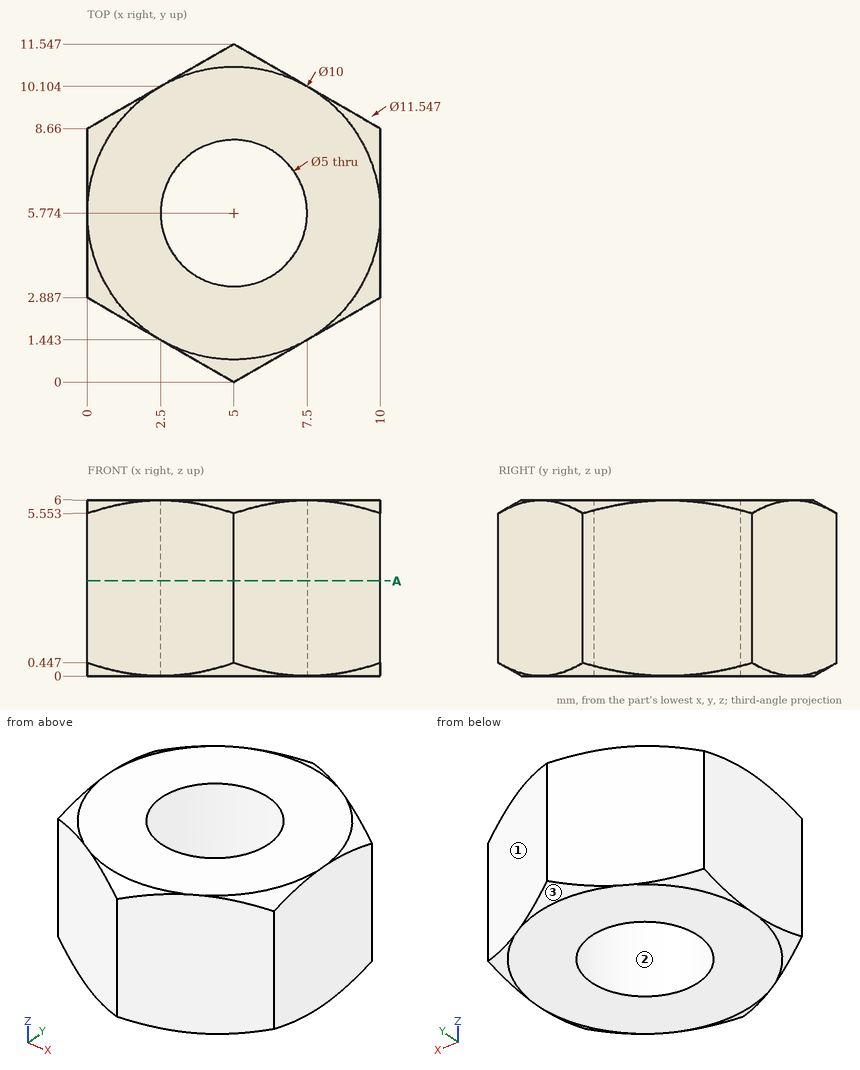
Drawing for the job (mm, zero at the part's lowest x, y, z). Give positions to 0.01 mm unless a question says otherwise; leave off trailing zeros. Write each loop counter-clockwise with the first axis right and the second up, starting at its lowest first coordinate (ties: lowest second). Pieces come first, ordered by that corner, then holes. Notation, with made-up numbers: (-23.5, 6.5) -> (31.5, 6.5) arc R20 cw to (31.5, 16.5) -> close; hole circle Ø11 at (-8.5, 11). An arc over 180 degrees is marked (long way). Put each result on its own line as item: value. Start each with the question number.
Item 1: Wall check: L1, parallel to X at y = 5.75, z = 2.2; L2, parallel to Y at x = 4.25, z = 2.25 (1 decimal); L3, parallel to Y at x = 3.75, z = 1.2 (1 decimal). Give the ranges that are in metal, low to high. Write a range as [from, to].
Item 2: Pull direction X, two halves, no side cores. Call the marked faces 1, 2 and 3: pulls with the +X half, pulls with the -X half, needs draft (parallel to the pull), parting line crosses it, or undercut.
Item 3: Cut at A-A (z = 3.25). List the corners of the cut face in (x, y).
Item 4: Pin check, flat tips, straight feed: pin 1 Ø1 at (x, z) = (8, 3) entering from +Y (1 decimal); pin 2 Ø3 at (x, z) = (8.5, 4.5) entering from -Y (1 decimal). Stop position of each tip, or through.
Answer list:
1. L1: x = [0, 2.5], [7.5, 10]
1. L2: y = [0.4, 3.4], [8.2, 11.1]
1. L3: y = [0.7, 3.6], [7.9, 10.8]
2. face 1: pulls with the +X half
2. face 2: undercut
2. face 3: parting line crosses it
3. outline: (0, 2.89) -> (5, 0) -> (10, 2.89) -> (10, 8.66) -> (5, 11.55) -> (0, 8.66) -> close; hole circle Ø5 at (5, 5.77)
4. pin 1: stops at y = 10.1
4. pin 2: stops at y = 1.2
